For this review, take the finished solid that the model builds, in its own axes (mm). Face numbers are marked on the shaded views. Coordinates: 2 decimals unless noted, no trailing zeros. Order: outer loops, then holes, each group sorted by start corner. A loop starts at its lowest first (then second) coordinate and runs counter-clockwise, first axis right, second up. Notation, with made-up numbers: (-13.5, -39) -> (11.5, -39) arc R20 ccw to (11.5, -22) -> close; hole circle Ø7 at (35.5, 33). An arc over 180 degrees is marked (long way). Write item = value, one per line. Start each with the question number.
1) Wall thickness on probe 1 along Y at (x, z) = (0, 12.75); probe 2 along Z at (x, y) = (0, -11) (1 decimal); probe 3 along Z at (x, y) = (7, -13): over which ranges is each line inside the solid? List them lowest first. Write a range as [from, to].
2) Consider section B-B on z = 0. Give the boundary of the cut face in (x, y) (1 decimal).
3) Insertion check: pin 1 Ø1 at (y, z) = (-7.5, 11.5) entering from +X; pin 2 Ø3 at (x, y) = (10, -13) entering from +Z; pin 3 Ø4 at (y, z) = (-4.5, 9.5) entering from -X; pin 4 Ø1 at (x, z) = (-9.5, 7.5) entering from +Y. Each pin has a flat end and moves straight along its axis. Give the tip position at first contact, or say it passes through.
4) Consider section A-A on x = 0. Give the boundary of the cut face in (y, z) (1 decimal), and give its area (3 significant figures).
5) Draft analysis for pull direction Z (two halves, no side actions). For the marked faces 1, 2 and 3, state which applies: +Z half, -Z half, draft (parallel to the pull), parting line (faces both ways), or undercut.
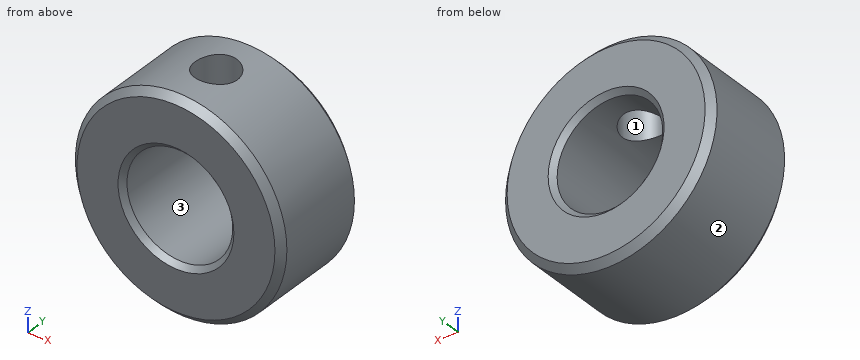
from build123d import *

# Parameters (mm, degrees)
F0_R     = 15.875
F0_R_2   = 7.9375
F1_DEPTH = 15.24
F2_SIZE  = 1.016
F3_SIZE  = 0.762
F5_R     = 3.175
F6_DEPTH = 14.224


with BuildPart() as f1:
    # F0 (on Front) → F1 (new body)
    with BuildSketch(Plane.XZ):
        Circle(F0_R)
        Circle(F0_R_2, mode=Mode.SUBTRACT)
    extrude(amount=F1_DEPTH)

    # F2
    f2_edges = [f1.edges().sort_by_distance(p)[0] for p in [
        (-15.875, -15.24, 0),
        (-15.875, 0, 0),
    ]]
    chamfer(f2_edges, length=F2_SIZE)

    # F3
    f3_edges = [f1.edges().sort_by_distance(p)[0] for p in [
        (-7.9375, -15.24, 0),
        (-7.9375, 0, 0),
    ]]
    chamfer(f3_edges, length=F3_SIZE)

    # F5 (on offset) → F6 (cut)
    with BuildSketch(Plane.XY.offset(15.875)):
        with Locations((0, -7.366)):
            Circle(F5_R)
    extrude(amount=-F6_DEPTH, mode=Mode.SUBTRACT)


solid = f1.part
Answer sheet:
q1.probe_1 = [-15.24, -10.54], [-4.19, 0]
q1.probe_2 = [-15.9, -7.9], [7.9, 15.9]
q1.probe_3 = [-14.25, -3.74], [3.74, 14.25]
q2.outline = (-15.9, -14.2) -> (-14.9, -15.2) -> (-8.7, -15.2) -> (-7.9, -14.5) -> (-7.9, -0.8) -> (-8.7, 0) -> (-14.9, 0) -> (-15.9, -1) -> close; (7.9, -14.5) -> (8.7, -15.2) -> (14.9, -15.2) -> (15.9, -14.2) -> (15.9, -1) -> (14.9, 0) -> (8.7, 0) -> (7.9, -0.8) -> close
q3.pin_1 = 11.45
q3.pin_2 = 13.41
q3.pin_3 = -13.99
q3.pin_4 = 0
q4.outline = (-15.2, -14.9) -> (-14.2, -15.9) -> (-1, -15.9) -> (0, -14.9) -> (0, -8.7) -> (-0.8, -7.9) -> (-14.5, -7.9) -> (-15.2, -8.7) -> close; (-15.2, 8.7) -> (-14.5, 7.9) -> (-10.5, 7.9) -> (-10.5, 15.9) -> (-14.2, 15.9) -> (-15.2, 14.9) -> close; (-4.2, 7.9) -> (-0.8, 7.9) -> (0, 8.7) -> (0, 14.9) -> (-1, 15.9) -> (-4.2, 15.9) -> close
q4.area = 188 mm2
q5.face_1 = draft
q5.face_2 = parting line
q5.face_3 = undercut
